Geometry: final body of the model. Coordinates: model frame, mm. Face numbers are marked on the shaded views. A direction names the side the tool comes from. Give positions to 0.01 mm unless a question says otherwise; leave off trailing zeros. Write each loop counter-clockwise with the first axis right and the second up, starting at its lowest first coordinate (ties: lowest second). Pieces come first, ordered by that corner, then holes. Notation, with made-up numbers: (-5, -16) -> (26, -16) arc R7 ccw to (26, -10) -> close; hole circle Ø6 at (86.25, 35). An arc over 180 degrees is marked (long way). Answer in a Markdown table with one row per item. Add a question column.
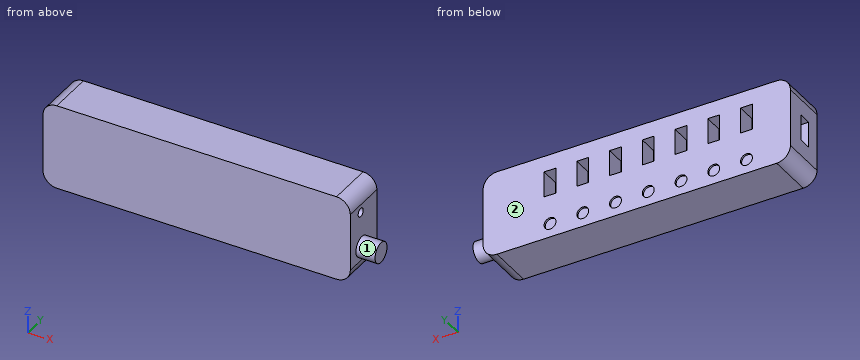
Autodesk Inventor part; units mm, degrees
ref_plane "YZ Plane" through (0, 0, 0) normal (1, 0, 0) x (0, 1, 0)
ref_plane "XZ Plane" through (0, 0, 0) normal (0, 1, 0) x (-1, 0, 0)
ref_plane "XY Plane" through (0, 0, 0) normal (0, 0, 1) x (1, 0, 0)
sketch "Sketch1" plane through (0, 0, 0) normal (0, 1, 0) x (-1, 0, 0)
  line L0 (0, 0) -> (-160.5, 0)
  line L1 (-160.5, 0) -> (-160.5, 44.5)
  line L2 (-160.5, 44.5) -> (0, 44.5)
  line L3 (0, 44.5) -> (0, 0)
  dimension "d0" = 44.5
  dimension "d1" = 160.5
extrude "Extrusion1" add sketch "Sketch1" along normal blind 23.6
fillet "Fillet1" radius 7.2 4 edges at (0, 11.8, 44.5) (160.5, 11.8, 44.5) (160.5, 11.8, 0) (0, 11.8, 0)
sketch "Sketch2" plane through (160.5, 0, 37.3) normal (1, 0, 0) x (0, 0, -1)
  circle A0 centre (4.15, 9.25) radius 2.25
  line L0 (-7.2, 23.6) -> (-7.2, 0)
  line L1 (6.4, 23.6) -> (6.4, 0) construction
  line L2 (0, 23.6) -> (30.1, 23.6) construction
  line L3 (30.1, 0) -> (0, 0) construction
  line L4 (13.7348, 11.5) -> (-5.9943, 11.5) construction
  line L5 (0, 0) -> (-7.2, 0) construction
  point P0 (37.3, 0)
  dimension "d5" = 4.5
  dimension "d7" = 13.6
  dimension "d8" = 11.5
extrude "Extrusion2" cut sketch "Sketch2" against normal blind 10
sketch "Sketch3" plane through (160.5, 0, 37.3) normal (1, 0, 0) x (0, 0, -1)
  circle A0 centre (23, 10.3) radius 5.3
  line L0 (17.7, 15.6) -> (17.7, 1.2331) construction
  line L1 (17.7, 15.6) -> (23.008, 15.6) construction
  line L2 (30.1, 0) -> (0, 0) construction
  line L3 (37.3, 0) -> (37.3, 23.6) construction
  dimension "d11" = 10.6
  dimension "d12" = 15.6
  dimension "d13" = 19.6
extrude "Extrusion3" add sketch "Sketch3" along normal blind 10
sketch "Sketch4" plane through (0, 0, 7.2) normal (-1, 0, 0) x (0, 0, 1)
  line L0 (8.3, 14.15) -> (21.8, 14.15)
  line L1 (21.8, 14.15) -> (21.8, 7.35)
  line L2 (21.8, 7.35) -> (8.3, 7.35)
  line L3 (8.3, 7.35) -> (8.3, 14.15)
  line L4 (30.1, 0) -> (0, 0)
  line L5 (-7.2, 23.6) -> (-7.2, 0)
  line L6 (37.3, 0) -> (37.3, 23.6)
  dimension "d16" = 7.35
  dimension "d17" = 6.8
  dimension "d18" = 13.5
  dimension "d19" = 15.5
  dimension "d20" = 15.5
extrude "Extrusion4" cut sketch "Sketch4" against normal blind 20
sketch "Sketch5" plane through (0, 23.6, 0) normal (0, 1, 0) x (1, 0, 0)
  line L0 (0.85, -43.7) -> (159.65, -43.7) construction
  line L1 (159.65, -43.7) -> (159.65, -0.8) construction
  line L2 (159.65, -0.8) -> (0.85, -0.8) construction
  line L3 (0.85, -0.8) -> (0.85, -43.7) construction
  line L4 (153.3, 0) -> (7.2, 0) construction
  line L5 (7.2, -44.5) -> (153.3, -44.5) construction
  line L6 (0, -7.2) -> (0, -37.3) construction
  line L7 (160.5, -37.3) -> (160.5, -7.2) construction
  line L8 (19.85, -36.15) -> (26.05, -36.15)
  line L9 (26.05, -36.15) -> (26.05, -22.65)
  line L10 (26.05, -22.65) -> (19.85, -22.65)
  line L11 (19.85, -22.65) -> (19.85, -36.15)
  line L12 (43.15, -36.15) -> (43.15, -22.65)
  line L13 (43.15, -22.65) -> (36.95, -22.65)
  line L14 (36.95, -22.65) -> (36.95, -36.15)
  line L15 (36.95, -36.15) -> (43.15, -36.15)
  line L16 (60.25, -36.15) -> (60.25, -22.65)
  line L17 (60.25, -22.65) -> (54.05, -22.65)
  line L18 (54.05, -22.65) -> (54.05, -36.15)
  line L19 (54.05, -36.15) -> (60.25, -36.15)
  line L20 (77.35, -36.15) -> (77.35, -22.65)
  line L21 (77.35, -22.65) -> (71.15, -22.65)
  line L22 (71.15, -22.65) -> (71.15, -36.15)
  line L23 (71.15, -36.15) -> (77.35, -36.15)
  line L24 (94.45, -36.15) -> (94.45, -22.65)
  line L25 (94.45, -22.65) -> (88.25, -22.65)
  line L26 (88.25, -22.65) -> (88.25, -36.15)
  line L27 (88.25, -36.15) -> (94.45, -36.15)
  line L28 (111.55, -36.15) -> (111.55, -22.65)
  line L29 (111.55, -22.65) -> (105.35, -22.65)
  line L30 (105.35, -22.65) -> (105.35, -36.15)
  line L31 (105.35, -36.15) -> (111.55, -36.15)
  line L32 (128.65, -36.15) -> (128.65, -22.65)
  line L33 (128.65, -22.65) -> (122.45, -22.65)
  line L34 (122.45, -22.65) -> (122.45, -36.15)
  line L35 (122.45, -36.15) -> (128.65, -36.15)
  point P0 (0, 0)
  dimension "d23" = 42.9
  dimension "d24" = 158.8
  dimension "d25" = 0.8
  dimension "d27" = 0.8
  dimension "d28" = 0.85
  dimension "d29" = 0.85
  dimension "d30" = 7.55
  dimension "d31" = 13.5
  dimension "d32" = 6.2
  dimension "d33" = 19
  dimension "d36" = 17.1
extrude "Extrusion5" cut sketch "Sketch5" against normal blind 10
sketch "Sketch6" plane through (0, 23.6, 0) normal (0, 1, 0) x (1, 0, 0)
  circle A0 centre (22.95, -7.3) radius 3.1
  line L0 (19.85, -36.15) -> (19.85, -22.65)
  line L1 (26.05, -22.65) -> (26.05, -36.15)
  line L2 (153.3, 0) -> (7.2, 0)
  circle A1 centre (40.05, -7.3) radius 3.1
  circle A2 centre (57.15, -7.3) radius 3.1
  circle A3 centre (74.25, -7.3) radius 3.1
  circle A4 centre (91.35, -7.3) radius 3.1
  circle A5 centre (108.45, -7.3) radius 3.1
  circle A6 centre (125.55, -7.3) radius 3.1
  point P0 (0, 0)
  dimension "d43" = 4.2
  dimension "d46" = 17.1
extrude "Extrusion6" cut sketch "Sketch6" against normal blind 1
equation "\"d20\" = d19"
equation "\"d27\" = d25"
equation "\"d29\" = d28"
properties part number "hub_dummy"
Q1. Section A-A on x = 74.25. Return loops of the section in (y, z), and give its area (3 significant figures).
Q2. Contact query for flat-ended pins moving along their axis: pin 1 Ø3 at (y, z) = (18, 27) entering from +X; pin 2 Ø1 at (y, z) = (5, 39.5) entering from -X; pin 3 Ø1.9 at (x, z) = (108.5, 6) entering from +Y; pin 4 Ø3 at (y, z) = (20.5, 28.5) entering from -X. Output: stop coordinate, or through.
Q3. Section B-B on z = 17. Return loops of the section in (x, y).
Q4. Line query: probe 1 along Z at (x, y) = (22.95, 23.35); probe 2 along Z at (x, y) = (89, 16.5); probe 3 along Y at (x, z) = (71.5, 25). Output: solid intervals per line, ascending. Write a range as from..to.
Q5. Access query for the marked faces 1 and 2. Directions: +Z, -Z, +X, -X, +Y, -Y. A direction counts if a zero-diameter tool reaches every point of the face in a straight line with its end or side. Return the directions, or none.
Q6. Section C-C on y = 20.5. Count the separate pieces of the cut face and the enclosed holes in it, and give its area (3 significant figures).
Checks:
| question | item | result |
|---|---|---|
| 1 | outline | (0, 0) -> (23.6, 0) -> (23.6, 4.2) -> (22.6, 4.2) -> (22.6, 10.4) -> (23.6, 10.4) -> (23.6, 22.65) -> (13.6, 22.65) -> (13.6, 36.15) -> (23.6, 36.15) -> (23.6, 44.5) -> (0, 44.5) -> close |
| 1 | area | 909 mm^2 |
| 2 | pin 1 | x = 160.5 |
| 2 | pin 2 | x = 0.2 |
| 2 | pin 3 | y = 22.6 |
| 2 | pin 4 | x = 0 |
| 3 | outline | (0, 0) -> (160.5, 0) -> (160.5, 5.74) -> (170.5, 5.74) -> (170.5, 14.86) -> (160.5, 14.86) -> (160.5, 23.6) -> (0, 23.6) -> (0, 14.15) -> (20, 14.15) -> (20, 7.35) -> (0, 7.35) -> close |
| 4 | probe 1 | 0..4.2, 10.4..22.65, 36.15..44.5 |
| 4 | probe 2 | 0..22.65, 36.15..44.5 |
| 4 | probe 3 | 0..13.6 |
| 5 | face 1 | +X |
| 5 | face 2 | +Z, -Z, +X, -X, +Y |
| 6 | separate pieces | 1 |
| 6 | enclosed holes | 7 |
| 6 | area | 6,510 mm^2 |
